Geometry: see drawing. Coordinates: mm, zero at the bounding-box minimum. A direction names the side the tool comes from. Round coordinates to 2 decimals unless told otherwise and drop trailing zeros. Loops run counter-clockwise (first coordinate to the right, second up) from the corner with the lowest first, then second, coordinate; pieces in that order, holes last. Notation, with made-up numbers: (20, 36.25) - (54, 36.25) arc R30 ccw to (54, 75.25) - close; hole circle Ø9 at (-32.5, 28.25). An arc over 180 degrees is marked (long way). Write item = value, one per line. Start each with the question number.
Item 1: Draft query along X for the marked faces 1, 2 and 3. Return one class per face: pulls with the +X half, pulls with the -X half, needs draft (parallel to the pull), parting line crosses it, or undercut.
Item 2: Section A-A (z = 15.5). Return loops of the section in (x, y) (3 decimals).
Item 3: Line query: line 1 (X direction, y = 18, z = 6) (3 decimals); line 2 (Y direction, x = 67.75, z = 38.1) (3 decimals); line 3 (Y direction, x = 51, z = 7.5) (3 decimals). Output: solid intervals per line, ascending. Write a range as from..to.
Item 4: Section C-C (x = 27.5). Return loops of the section in (y, z) (3 decimals), plus the area to 3 significant figures.
Item 5: Section D-D (y = 35.5). Return loops of the section in (x, z) (3 decimals).
Item 6: Access query for the marked faces 4 and 5. Directions: +Z, -Z, +X, -X, +Y, -Y. A direction counts if a zero-diameter tool reaches every point of the face in a straight line with its end or side. Return the directions, or none.
Item 7: First-contact query: pin 1 (1.5 mm diameter, centred on x = 9, z = 16.5, fed in from +Y) (3 decimals). Flat tip, straight axial feed; report the tip coordinate or a pass-through.
Item 8: Section B-B (y = 10). Return loops of the section in (x, z) (3 decimals).
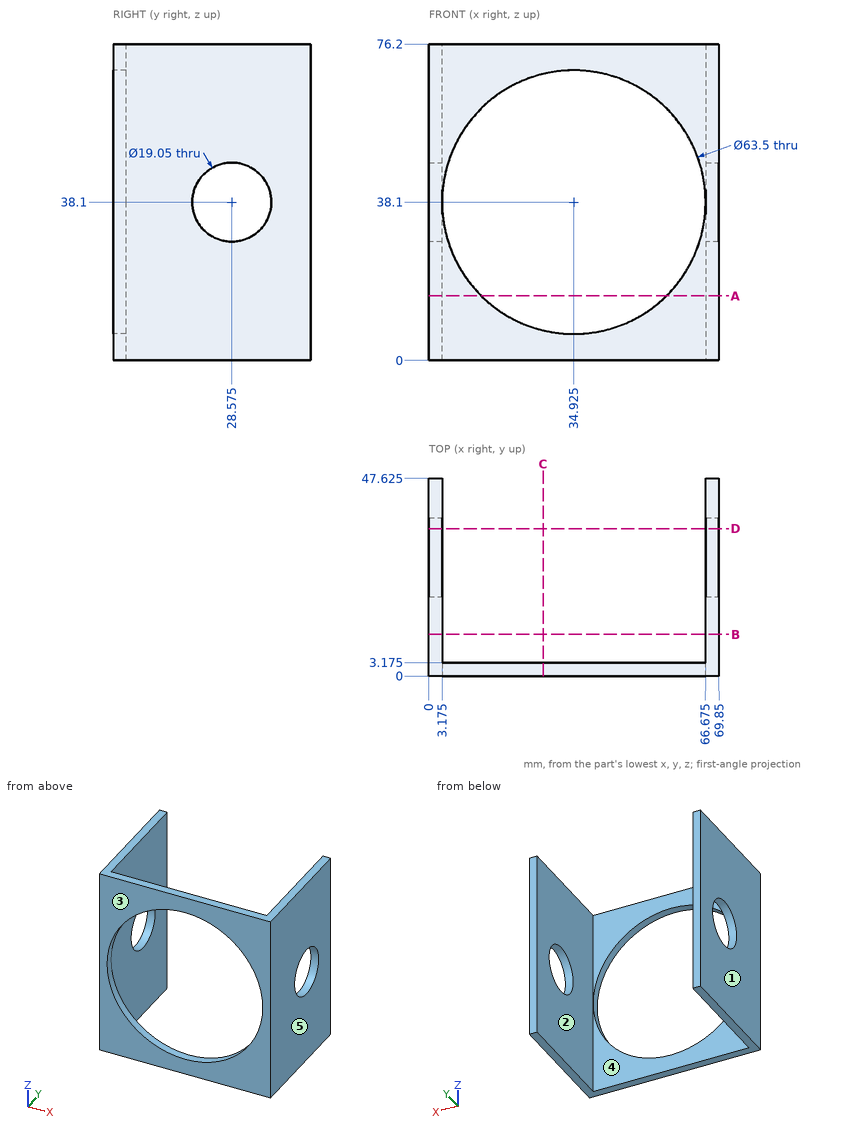
Taken from the geometry:
q1.face_1 = pulls with the -X half
q1.face_2 = undercut
q1.face_3 = needs draft
q2.outline = (0, 0) - (12.625, 0) - (12.625, 3.175) - (3.175, 3.175) - (3.175, 47.625) - (0, 47.625) - close; (57.225, 0) - (69.85, 0) - (69.85, 47.625) - (66.675, 47.625) - (66.675, 3.175) - (57.225, 3.175) - close
q3.line_1 = 0..3.175, 66.675..69.85
q3.line_2 = 0..19.05, 38.1..47.625
q3.line_3 = 0..3.175
q4.outline = (0, 0) - (3.175, 0) - (3.175, 7.23) - (0, 7.23) - close; (0, 68.97) - (3.175, 68.97) - (3.175, 76.2) - (0, 76.2) - close
q4.area = 45.9 mm^2
q5.outline = (0, 0) - (3.175, 0) - (3.175, 31.56) - (0, 31.56) - close; (0, 44.64) - (3.175, 44.64) - (3.175, 76.2) - (0, 76.2) - close; (66.675, 0) - (69.85, 0) - (69.85, 31.56) - (66.675, 31.56) - close; (66.675, 44.64) - (69.85, 44.64) - (69.85, 76.2) - (66.675, 76.2) - close
q6.face_4 = +Z, -Z, +Y
q6.face_5 = +Z, -Z, +X, +Y, -Y
q7.pin_1 = 3.175
q8.outline = (0, 0) - (3.175, 0) - (3.175, 76.2) - (0, 76.2) - close; (66.675, 0) - (69.85, 0) - (69.85, 76.2) - (66.675, 76.2) - close
